Check sheet for the drawn part. Datum: minimum x, y, z corner. Units: mm. Round coordinates to 2 decimals unless told otherwise and drop trailing zeros. Write each loop counter-clockwise with the first axis right and the second up, starting at its lowest first coordinate (ties: lowest second). Pieces come first, ordered by that corner, then holes. Notation, with made-up numbers: (66, 29) -> (82, 29) arc R19 ccw to (82, 55) -> close; hole circle Ø9 at (63.25, 12). An arc over 180 degrees is marked (long way). One line per item, written item: value. Start each with the question number.
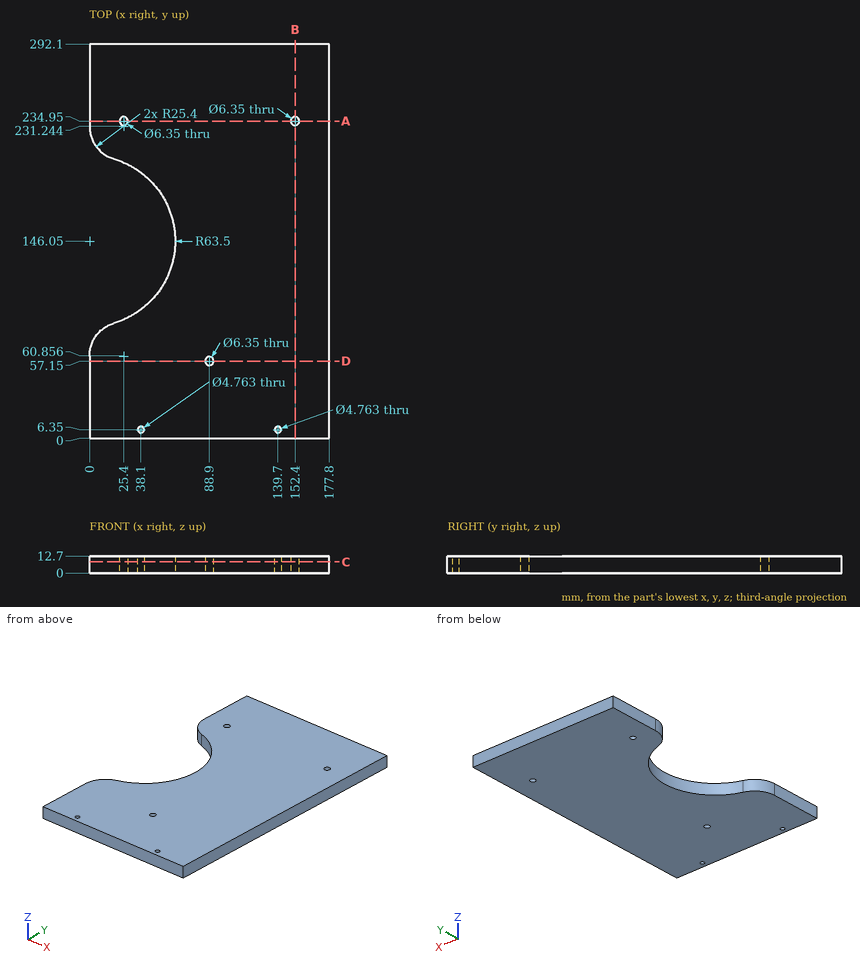
1. Depth check by flat-ended pin: pin 1 Ø4 at (x, y) = (88.9, 57.15) entering from -Z; pin 2 Ø5 at (y, z) = (93, 10.5) entering from -X (1 decimal). Enter the tip coordinate at first touch or a pass-through.
2. Cross-section at B-B (x = 152.4). Record the cut outline in (y, z) (1 decimal).
3. Cross-section at A-A (y = 234.95). Record the cut outline in (x, z) (1 decimal), plus the area to 3 significant figures.
4. Cross-section at C-C (z = 8.5). Give the number of separate pieces and of enclosed holes in the cut face, plus the area to 3 significant figures.
5. Material ranges on probe 1 along X at (y, z) = (235.5, 1); probe 2 along Y at (x, z) = (152.4, 6.25) (1 decimal); probe 3 along X at (y, z) = (59.5, 0.5) (1 decimal), recorded low to high.
6. Cross-section at D-D (y = 57.15). Record the cut outline in (x, z) (1 decimal).
Working result:
1. pin 1: passes through
1. pin 2: stops at x = 30.8
2. outline: (0, 0) -> (231.8, 0) -> (231.8, 12.7) -> (0, 12.7) -> close; (238.1, 0) -> (292.1, 0) -> (292.1, 12.7) -> (238.1, 12.7) -> close
3. outline: (0, 0) -> (22.2, 0) -> (22.2, 12.7) -> (0, 12.7) -> close; (28.6, 0) -> (149.2, 0) -> (149.2, 12.7) -> (28.6, 12.7) -> close; (155.6, 0) -> (177.8, 0) -> (177.8, 12.7) -> (155.6, 12.7) -> close
3. area: 2,100 mm^2
4. separate pieces: 1
4. enclosed holes: 5
4. area: 45,300 mm^2
5. probe 1: x = 0 to 22.27, 28.53 to 149.27, 155.53 to 177.8
5. probe 2: y = 0 to 231.8, 238.1 to 292.1
5. probe 3: x = 0 to 86.8, 91 to 177.8
6. outline: (0, 0) -> (85.7, 0) -> (85.7, 12.7) -> (0, 12.7) -> close; (92.1, 0) -> (177.8, 0) -> (177.8, 12.7) -> (92.1, 12.7) -> close
